Input: dimensioned drawing with shaded views. Units: mm. Origin: part minimum x, y, z. A direction names the side the tool comes from. Round coordinates to 2 decimals unless told otherwise and drop trailing zeros. Loops run counter-clockwise (first coordinate to the right, second up) from the corner with the lowest first, then second, coordinate; pieces in that order, holes last.
Item 1: Section query A-A on x = 0.2. Return loops of the section in (y, z).
Item 2: Access query for the marked faces 4 and 5. Directions: +Z, -Z, +X, -X, +Y, -Y. A direction counts if a zero-diameter tool reaches every point of the face in a straight line with its end or side. Return the directions, or none.
Item 3: Pull-direction query (Y, two-part tool) for the marked faces 1, 2 and 3; classes: released by +Y, released by -Y, zero draft, split by the parting line, or undercut.
Item 4: Ray query, L1, parallel to Z at x = 0.75, y = 4.1; L2, parallel to Y at x = 0.55, z = 4.25; L3, parallel to Y at x = 0.4, z = 9. Return the intervals inside material, ascending.
Item 5: Section query B-B on y = 3.7. Return loops of the section in (x, z), then the cut area to 3 significant figures.
Item 6: Section query C-C on z = 9. Return loops of the section in (x, y).
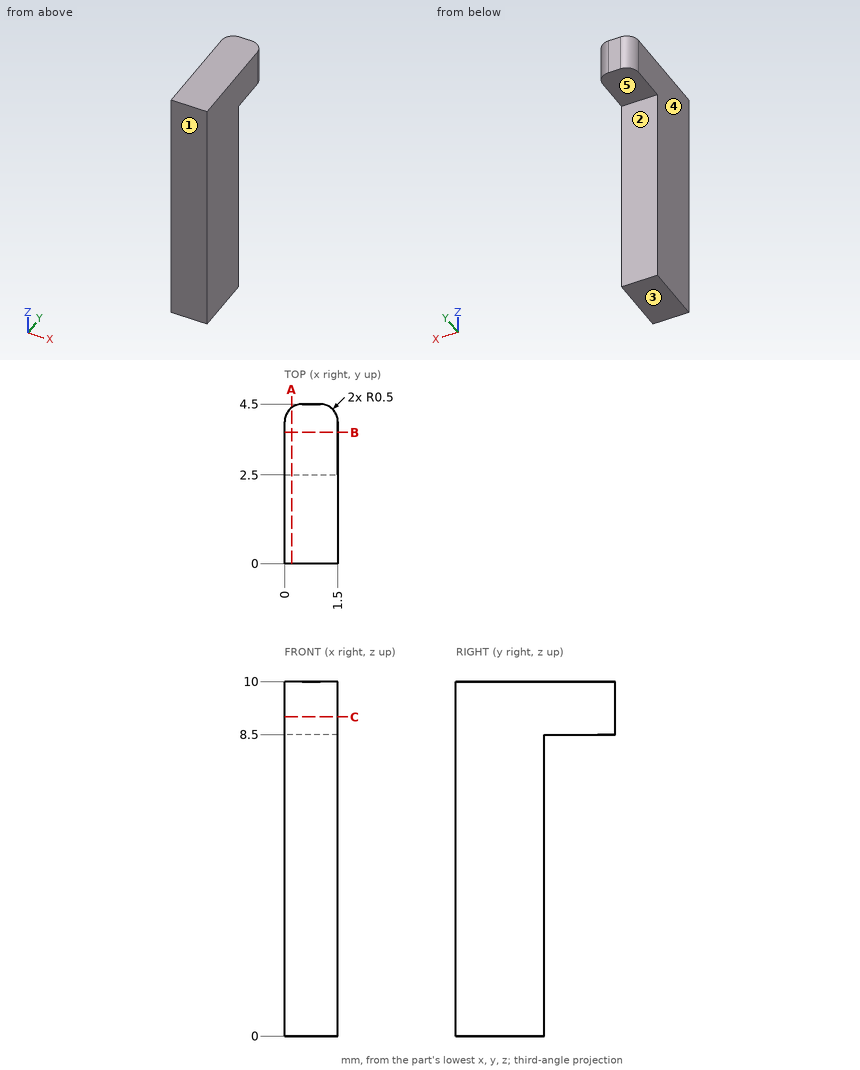
Data:
1. outline: (0, 0) - (2.5, 0) - (2.5, 8.5) - (4.4, 8.5) - (4.4, 10) - (0, 10) - close
2. face 4: +Z, -Z, -X, +Y, -Y
2. face 5: -Z, +X, -X, +Y
3. face 1: released by -Y
3. face 2: released by +Y
3. face 3: zero draft
4. L1: z = 8.5 to 10
4. L2: y = 0 to 2.5
4. L3: y = 0 to 4.49
5. outline: (0, 8.5) - (1.5, 8.5) - (1.5, 10) - (0, 10) - close
5. area: 2.25 mm2
6. outline: (0, 0) - (1.5, 0) - (1.5, 4) arc R0.5 ccw to (1, 4.5) - (0.5, 4.5) arc R0.5 ccw to (0, 4) - close
